from build123d import *

# Parameters (mm, degrees)
BOSS_EXTRUDE1_DEPTH = 10
DRAFT1_ANGLE        = 45
BOSS_EXTRUDE2_DEPTH = 30
SKETCH6_W           = 50
SKETCH6_H           = 17.7
BOSS_EXTRUDE3_DEPTH = 50
SKETCH7_W           = 50
SKETCH7_H           = 7.7
CUT_EXTRUDE4_DEPTH  = 20


with BuildPart() as part:
    # Sketch2 → Boss-Extrude1 (new body)
    with BuildSketch(Plane(origin=(0, 0, 0), x_dir=(1, 0, 0), z_dir=(0, 1, 0))):
        Polygon((-90, 5), (90, 5), (120, -55), (115.527864045, -57.236067977), (88.291796068, -2.763932023), (-88.291796068, -2.763932023), (-115.527864045, -57.236067977), (-120, -55), align=None)
    extrude(amount=BOSS_EXTRUDE1_DEPTH)

    # Draft1
    draft1_faces = [part.faces().sort_by_distance(p)[0] for p in [
        (101.909830056, 5, 30),
        (0, 5, 2.763932023),
        (-101.909830056, 5, 30),
    ]]
    draft(draft1_faces, Plane.ZX.offset(10), DRAFT1_ANGLE)

    # Sketch5 → Boss-Extrude2 (add)
    with BuildSketch(Plane(origin=(0, 10, 0), x_dir=(1, 0, 0), z_dir=(0, 1, 0))):
        Polygon((-120, -55), (-90, 5), (90, 5), (120, -55), (115.527864045, -57.236067977), (88.291796068, -2.763932023), (-88.291796068, -2.763932023), (-115.527864045, -57.236067977), align=None)
    extrude(amount=BOSS_EXTRUDE2_DEPTH)

    # Sketch6 → Boss-Extrude3 (add)
    with BuildSketch(Plane(origin=(0, 0, -5), x_dir=(-1, 0, 0), z_dir=(0, 0, -1))):
        with Locations((0, 14.45)):
            Rectangle(SKETCH6_W, SKETCH6_H)
    extrude(amount=BOSS_EXTRUDE3_DEPTH)

    # Sketch7 → Cut-Extrude4 (cut)
    with BuildSketch(Plane(origin=(0, 0, -55), x_dir=(-1, 0, 0), z_dir=(0, 0, -1))):
        with Locations((0, 14.45)):
            Rectangle(SKETCH7_W, SKETCH7_H)
    extrude(amount=-CUT_EXTRUDE4_DEPTH, mode=Mode.SUBTRACT)


solid = part.part
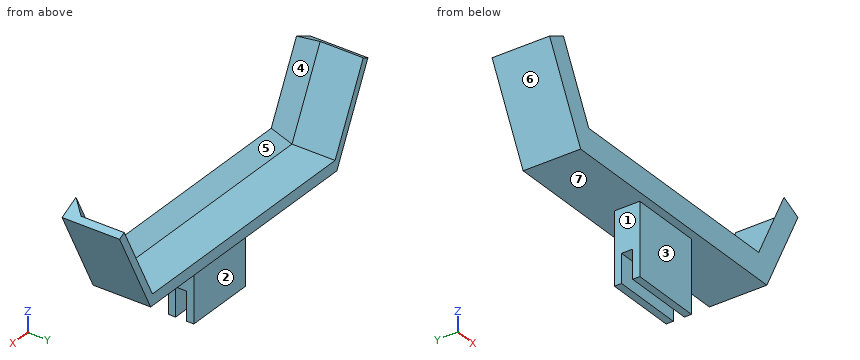
CAD build for the part. Positions are in the model's coordinates, mm. Face numbers are marked on the shaded views. A direction names the side the tool comes from. Give positions to 0.01 mm unless a question says otherwise; leave off trailing zeros. Order: outer loops, then holes, each group sorted by start corner. A loop starts at its lowest first (then second) coordinate and runs counter-clockwise, first axis right, second up. Notation, with made-up numbers: (-21, 78) - (36, 78) arc R9 ccw to (36, 84) - close; hole circle Ø2 at (58.25, 57). An arc over 180 degrees is marked (long way). Answer in a Markdown table with one row per item.
1. Flat gauge pins, fed straight in: pin 1 (6 mm diameter, centred on x = -7.5, z = -47.5, fed in from -Y); pin 2 (19.5 mm diameter, centred on y = 14, z = -24.5, fed in from -X); pin 3 (15 mm diameter, centred on x = 4, z = -21.5, fed in from +Y); pin 4 (6 mm diameter, centred on x = 8, y = 13, fed in from -Z). Where does each tip first touch, or does it go through?
Data:
| item | result |
|---|---|
| pin 1 | stops at y = 5.6 |
| pin 2 | stops at x = -25 |
| pin 3 | stops at y = 23.3 |
| pin 4 | stops at z = -55 |
2. Saw through at A-A, the plane z = -39.5. Give the cut face in (x, y).
Data:
| item | result |
|---|---|
| outline | (-25, 5.6) - (25, 5.6) - (25, 10.6) - (-25, 10.6) - close; (-25, 18.3) - (25, 18.3) - (25, 23.3) - (-25, 23.3) - close |
3. Tool access for the marked faces 1, 2, 3 and 4: list every direction of +Z, -Z, +X, -X, +Y, -Y with a clear straight run to the whole face (end or side of a thin tool).
Data:
| item | result |
|---|---|
| face 1 | -Z, -X, +Y, -Y |
| face 2 | -Z, +X, -X, +Y |
| face 3 | -Z, +X, -X, -Y |
| face 4 | +Z, +Y |
4. Saw through at B-B, the plane y = 31. Give the cut face in (x, z), plus the area to 3 significant figures.
Data:
| item | result |
|---|---|
| outline | (-120, 55) - (-90, -5) - (90, -5) - (120, 55) - (115.53, 57.24) - (88.29, 2.76) - (-88.29, 2.76) - (-115.53, 57.24) - close |
| area | 2,020 mm² |
5. Pull direction X, two halves, no side cores. Call the marked faces 5, 6 and 7: pulls with the +X half, pulls with the -X half, needs draft (parallel to the pull), parting line crosses it, or undercut.
Data:
| item | result |
|---|---|
| face 5 | undercut |
| face 6 | pulls with the -X half |
| face 7 | needs draft |
6. Saw through at D-D, the plane z = 43.5. Give the cut face in (x, y), plus the area to 3 significant figures.
Data:
| item | result |
|---|---|
| outline | (-114.25, 0) - (-97.48, 0) - (-108.66, 10) - (-108.66, 40) - (-114.25, 40) - close; (97.48, 0) - (114.25, 0) - (114.25, 40) - (108.66, 40) - (108.66, 10) - close |
| area | 559 mm² |
7. Probe probe 1 along Y at (x, z) = (-9.5, -38.5); probe 2 along Z at (x, y) = (16.5, 23); probe 3 along X at (y, z) = (30.5, 42.5). List the from-to ranges inside material, lowest first. Write a range as [from, to].
Data:
| item | result |
|---|---|
| probe 1 | y = [5.6, 10.6], [18.3, 23.3] |
| probe 2 | z = [-55, 2.76] |
| probe 3 | x = [-113.75, -108.16], [108.16, 113.75] |
8. Saw through at C-C, the plane x = 74. Give the cut face in (y, z).
Data:
| item | result |
|---|---|
| outline | (0, -5) - (40, -5) - (40, 2.76) - (10, 2.76) - (0, 12.76) - close |
